from build123d import *

# Parameters (mm, degrees)
SKETCH2_W           = 65
SKETCH2_H           = 30
BOSS_EXTRUDE1_DEPTH = 5
SKETCH3_R           = 1.6
CUT_EXTRUDE1_DEPTH  = 37.142080737
SKETCH5_W           = 30
SKETCH5_H           = 5
BOSS_EXTRUDE2_DEPTH = 7.5
CUT_EXTRUDE2_DEPTH  = 10


with BuildPart() as part:
    # Sketch2 → Boss-Extrude1 (new body)
    with BuildSketch(Plane(origin=(0, 0, 0), x_dir=(1, 0, 0), z_dir=(0, 1, 0))):
        Rectangle(SKETCH2_W, SKETCH2_H)
    extrude(amount=BOSS_EXTRUDE1_DEPTH)

    # Sketch3 → Cut-Extrude1 (cut, through all)
    with BuildSketch(Plane(origin=(0, 5, 0), x_dir=(1, 0, 0), z_dir=(0, 1, 0))):
        with Locations(Location((-27.5, 0, 0), (0, 0, 270))):
            Circle(SKETCH3_R)
        with Locations(Location((-18, 9.5, 0), (0, 0, 270))):
            Circle(SKETCH3_R)
        with Locations(Location((-8.5, 0, 0), (0, 0, 270))):
            Circle(SKETCH3_R)
        with Locations(Location((-18, -9.5, 0), (0, 0, 270))):
            Circle(SKETCH3_R)
        with Locations(Location((18, -9.5, 0), (0, 0, 90))):
            Circle(SKETCH3_R)
        with Locations(Location((27.5, 0, 0), (0, 0, 90))):
            Circle(SKETCH3_R)
        with Locations(Location((18, 9.5, 0), (0, 0, 90))):
            Circle(SKETCH3_R)
        with Locations(Location((8.5, 0, 0), (0, 0, 90))):
            Circle(SKETCH3_R)
    extrude(amount=-CUT_EXTRUDE1_DEPTH, mode=Mode.SUBTRACT)

    # Sketch5 → Boss-Extrude2 (add)
    with BuildSketch(Plane(origin=(32.5, 0, 0), x_dir=(0, 0, -1), z_dir=(1, 0, 0))):
        with Locations((0, 2.5)):
            Rectangle(SKETCH5_W, SKETCH5_H)
    extrude(amount=BOSS_EXTRUDE2_DEPTH)

    # Sketch4 → Cut-Extrude2 (cut)
    with BuildSketch(Plane(origin=(0, 5, 0), x_dir=(1, 0, 0), z_dir=(0, 1, 0))):
        with BuildLine():
            Line((8.5, 1.6), (16, 1.6))
            ThreePointArc((16, 1.6), (17.6, 0), (16, -1.6))
            Line((16, -1.6), (8.5, -1.6))
            ThreePointArc((8.5, -1.6), (6.9, 0), (8.5, 1.6))
        make_face()
        with BuildLine():
            Line((27.5, 1.6), (35, 1.6))
            ThreePointArc((35, 1.6), (36.6, 0), (35, -1.6))
            Line((35, -1.6), (27.5, -1.6))
            ThreePointArc((27.5, -1.6), (25.9, 0), (27.5, 1.6))
        make_face()
        with BuildLine():
            Line((18, -7.9), (25.5, -7.9))
            ThreePointArc((25.5, -7.9), (27.1, -9.5), (25.5, -11.1))
            Line((25.5, -11.1), (18, -11.1))
            ThreePointArc((18, -11.1), (16.4, -9.5), (18, -7.9))
        make_face()
        with BuildLine():
            Line((18, 11.1), (25.5, 11.1))
            ThreePointArc((25.5, 11.1), (27.1, 9.5), (25.5, 7.9))
            Line((25.5, 7.9), (18, 7.9))
            ThreePointArc((18, 7.9), (16.4, 9.5), (18, 11.1))
        make_face()
    extrude(amount=-CUT_EXTRUDE2_DEPTH, mode=Mode.SUBTRACT)


solid = part.part
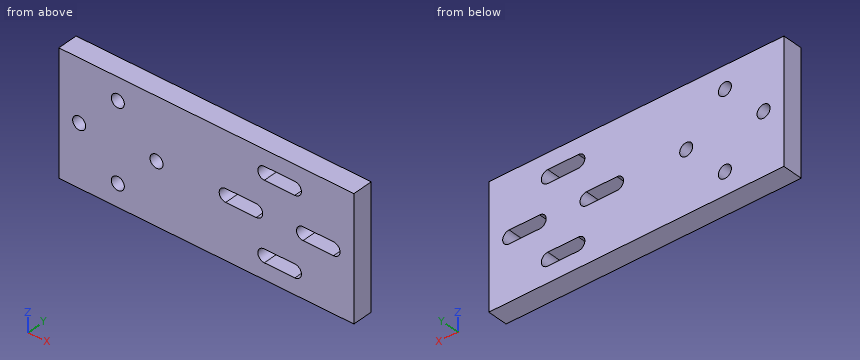
Check sheet for the modelled part. Datum: model origin and axes. Units: mm. Give positions to 0.01 mm unless a question says otherwise; leave off trailing zeros. Loops run counter-clockwise (first coordinate to the right, second up) from the corner with the lowest first, then second, coordinate; pieces in that order, holes last. Notation, with made-up numbers: M 72,68.25 L 113,68.25 A22 ccw 113,86.25 Z; hole C -20,40.25 d4. An arc over 180 degrees is marked long. Use a Markdown table: item, result. Add a question column.
Q1. Sectioned sample at C-C, the plane y = 1.7. Give the number of separate pieces and of enclosed holes in the cut face, then the cut area to 3 significant figures.
Q2. Sectioned sample at A-A, the plane z = 9.5. Record the cut outline in (x, y).
Q3. Go/stop test with flat-tipped pins: pin 1 (5 mm diameter, centred on x = -18, z = 9.5, fed in from +Y); pin 2 (1.9 mm diameter, centred on x = -18, z = -9.5, fed in from -Y). Record where each tip stops, or that it passes through.
Q4. Sectioned sample at B-B, the plane x = 13. Record the cut outline in (y, z), then the cut area to 3 significant figures.
Q5. Sectioned sample at D-D, the plane z = -10. Record the cut outline in (x, y), then the cut area to 3 significant figures.
Q6. Scan lines: line 1 along X through (y, z) = (1.7, -9.5); line 2 along X through (y, z) = (1.6, 0); line 3 along Z through (x, y) = (20.5, 2.3). Record each from-to range of solid material in increasing order. Write a range as [from, to].
Verdict:
| question | item | result |
|---|---|---|
| 1 | separate pieces | 1 |
| 1 | enclosed holes | 8 |
| 1 | area | 2,010 mm^2 |
| 2 | outline | M -32.5,0 L -19.6,0 L -19.6,5 L -32.5,5 Z; M -16.4,0 L 16.4,0 L 16.4,5 L -16.4,5 Z; M 27.1,0 L 40,0 L 40,5 L 27.1,5 Z |
| 3 | pin 1 | y = 5 |
| 3 | pin 2 | through |
| 4 | outline | M 0,-15 L 5,-15 L 5,-1.6 L 0,-1.6 Z; M 0,1.6 L 5,1.6 L 5,15 L 0,15 Z |
| 4 | area | 134 mm^2 |
| 5 | outline | M -32.5,0 L -19.52,0 L -19.52,5 L -32.5,5 Z; M -16.48,0 L 16.48,0 L 16.48,5 L -16.48,5 Z; M 27.02,0 L 40,0 L 40,5 L 27.02,5 Z |
| 5 | area | 295 mm^2 |
| 6 | line 1 | [-32.5, -19.6], [-16.4, 16.4], [27.1, 40] |
| 6 | line 2 | [-32.5, -29.1], [-25.9, -10.1], [-6.9, 6.9], [17.6, 25.9], [36.6, 40] |
| 6 | line 3 | [-15, -11.1], [-7.9, 7.9], [11.1, 15] |
